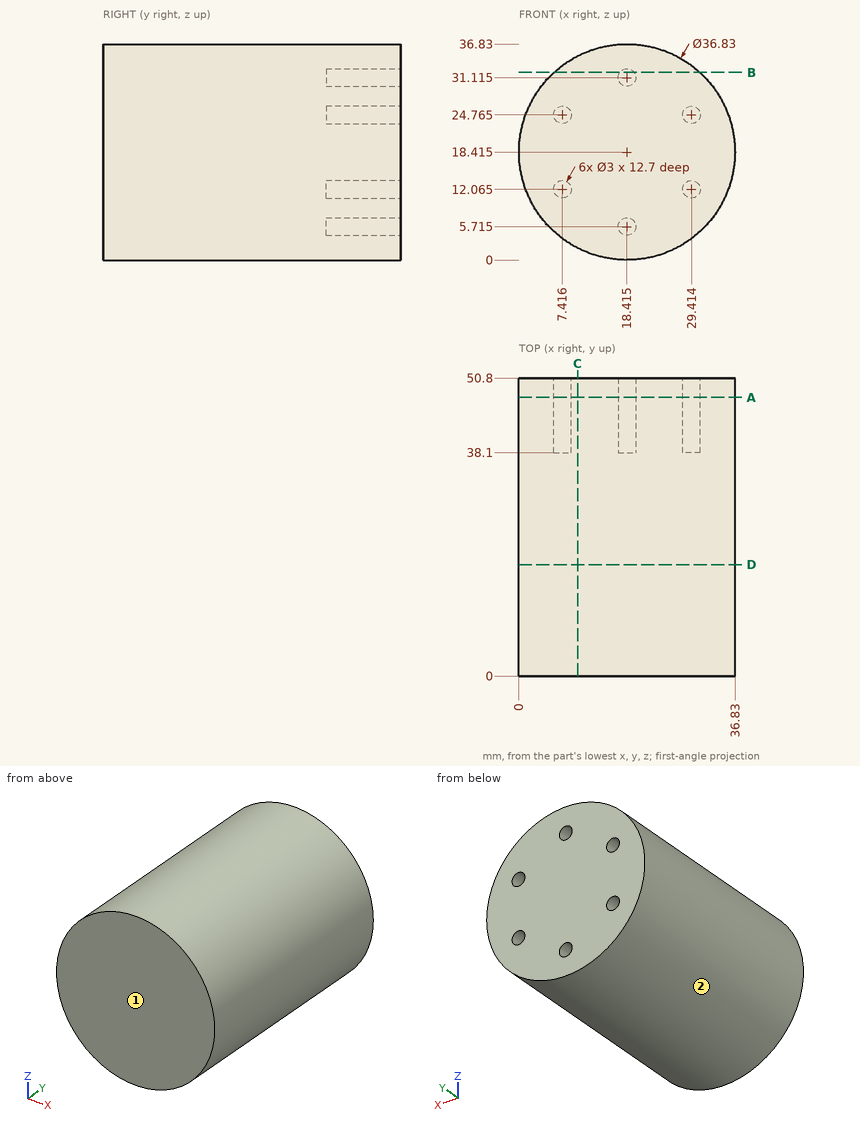
Here's the drawing with two shaded views (mm, measured from the low corner). I have some questions. Give positions to 0.01 mm unless a question says otherwise; leave off trailing zeros. Write each loop counter-clockwise with the first axis right and the second up, starting at its lowest first coordinate (ties: lowest second). Pieces come first, ordered by that corner, then holes. Notation, with made-up numbers: (-19, 5) - (39, 5) arc R16 cw to (39, 33) - close; hole circle Ø6 at (51, 21). An arc over 180 degrees is marked (long way). One line per item, written item: value. Start each with the question number.
Item 1: Please list where these lines run through material, in increasing order: line 1 (Z direction, x = 28.5, y = 42.5) (1 decimal); line 2 (X direction, y = 39, z = 25) (1 decimal); line 3 (X direction, y = 43, z = 31). Write a range as from..to.
Item 2: Imagine slicing it at D-D, the plane y = 19. List the corners of the cut face in (x, z) for me (1 decimal).
Item 3: If we mould it in two halves opening along X, with no side actions, what happens to the marked faces 1 and 2? For each: +X half, -X half, draft (parallel to the pull), parting line (faces both ways), or undercut.
Item 4: I'm going to push flat-ended pins straight in: pin 1 (2 mm diameter, centred on y = 25.5, z = 30.5, fed in from +X); pin 2 (1.5 mm diameter, centred on x = 6.5, z = 25, fed in from +Y); pin 3 (10 mm diameter, centred on y = 37.5, z = 31, fed in from +X) (1 decimal); pin 4 (0.9 mm diameter, centred on x = 18, z = 6, fed in from +Y). Where does each tip first touch, or does it pass through?
Item 5: Imagine slicing it at A-A, the plane y = 47.5. List the corners of the cut face in (x, z) for me (1 decimal), and give its area (3 significant figures).
Item 6: Imagine slicing it at B-B, the plane z = 32. List the corners of the cut face in (x, y) for me.
Item 7: Imagine slicing it at C-C, the plane x = 10. List the corners of the cut face in (y, z) for me (1 decimal).
Geometry says:
1. line 1: 3..10.9, 13.3..23.6, 26..33.8
1. line 2: 1.2..5.9, 8.9..27.9, 30.9..35.6
1. line 3: 4.97..16.92, 19.91..31.86
2. outline: circle Ø36.8 at (18.4, 18.4)
3. face 1: draft
3. face 2: parting line
4. pin 1: x = 33.12
4. pin 2: y = 50.8
4. pin 3: x = 35.2
4. pin 4: y = 38.1
5. outline: circle Ø36.8 at (18.4, 18.4); hole circle Ø3 at (7.4, 12.1); hole circle Ø3 at (7.4, 24.8); hole circle Ø3 at (18.4, 5.7); hole circle Ø3 at (18.4, 31.1); hole circle Ø3 at (29.4, 12.1); hole circle Ø3 at (29.4, 24.8)
5. area: 1,020 mm^2
6. outline: (5.98, 0) - (30.85, 0) - (30.85, 50.8) - (19.63, 50.8) - (19.63, 38.1) - (17.2, 38.1) - (17.2, 50.8) - (5.98, 50.8) - close
7. outline: (0, 2) - (50.8, 2) - (50.8, 34.8) - (0, 34.8) - close
